```python
from build123d import *

# Parameters (mm, degrees)
F0_W     = 177.8
F0_H     = 228.6
F0_W_2   = 165.1
F0_H_2   = 215.9
F1_DEPTH = 279.4
F2_R     = 12.7
F2_R_2   = 38.829729
F3_DEPTH = 254
F4_R     = 17.145
F5_DEPTH = 254
F6_DEPTH = 25.4


with BuildPart() as f1:
    # F0 (on Top) → F1 (new body)
    with BuildSketch(Plane.XY):
        Rectangle(F0_W, F0_H)
        Rectangle(F0_W_2, F0_H_2, mode=Mode.SUBTRACT)
    extrude(amount=F1_DEPTH)

    # F2 (on Front) → F3 (cut)
    with BuildSketch(Plane.XZ):
        with Locations((0, 80.557629)):
            Circle(F2_R)
        with Locations((0, 161.839798)):
            Circle(F2_R_2)
    extrude(amount=F3_DEPTH, mode=Mode.SUBTRACT)

    # F4 (on Right) → F5 (cut)
    with BuildSketch(Plane.YZ):
        with Locations((0, 101.838969)):
            Circle(F4_R)
    extrude(amount=F5_DEPTH, mode=Mode.SUBTRACT)

    # F0 (on Top) → F6 (join)
    with BuildSketch(Plane.XY):
        Rectangle(F0_W_2, F0_H_2)
    extrude(amount=F6_DEPTH)


solid = f1.part
```
The model under review builds one solid part; all positions refer to its coordinate system, in mm. A direction names the side the tool comes from. Round coordinates to 2 decimals unless told otherwise and drop trailing zeros. Loops run counter-clockwise (first coordinate to the right, second up) from the corner with the lowest first, then second, coordinate; pieces in that order, holes last. Notation, with made-up numbers: (3.25, 28) -> (62.25, 28) arc R12 cw to (62.25, 48) -> close; hole circle Ø9 at (72, -7.5). An arc over 180 degrees is marked (long way). Answer in a Markdown table with one row per item.
1) Tool access review of faces 1 (the flat face through (-1, -114.3, 107)), 2 (the cylindrical face through (-2.75, -111.08, 68.16)), 3 (the flat face through (-1, -107.95, 122)): name each direction out of +Z, -Z, +X, -X, +Y, -Y from which nothing blocks a thin tool from reaching the whole face with its end or side.
Taken from the geometry:
| item | result |
|---|---|
| face 1 | +Z, -Z, +X, -X, -Y |
| face 2 | -Y |
| face 3 | +Z |
2) Draft analysis for pull direction X (two halves, no side actions). For faces 4 (the flat face through (-88.9, -2, 138)), 5 (the cylindrical face through (85.68, -2.23, 118.84)), 6 (the flat face through (-1, 107.95, 151)), state which applies: pulls with the +X half, pulls with the -X half, needs draft (parallel to the pull), parting line crosses it, or undercut.
Taken from the geometry:
| item | result |
|---|---|
| face 4 | pulls with the -X half |
| face 5 | needs draft |
| face 6 | undercut |
3) Consider section A-A, the plane y = 0. Write out the cut boundary in (x, z).
Taken from the geometry:
| item | result |
|---|---|
| outline | (-88.9, 0) -> (88.9, 0) -> (88.9, 84.69) -> (82.55, 84.69) -> (82.55, 25.4) -> (-82.55, 25.4) -> (-82.55, 279.4) -> (-88.9, 279.4) -> close; (82.55, 118.98) -> (88.9, 118.98) -> (88.9, 279.4) -> (82.55, 279.4) -> close |
4) Wall thickness on line 1 along Z through (x, y) = (0, -112.25); line 2 along X through (y, z) = (-8.5, 225); line 3 along Y through (x, z) = (15, 237): over which ranges is each line inside the solid? List them lowest first.
Taken from the geometry:
| item | result |
|---|---|
| line 1 | z = 0 to 67.86, 93.26 to 123.01, 200.67 to 279.4 |
| line 2 | x = -88.9 to -82.55, 82.55 to 88.9 |
| line 3 | y = -114.3 to -107.95, 107.95 to 114.3 |
5) Consider section C-C, the plane z = 219.5. Write out the cut boundary in (x, y).
Taken from the geometry:
| item | result |
|---|---|
| outline | (-88.9, -114.3) -> (88.9, -114.3) -> (88.9, 114.3) -> (-88.9, 114.3) -> close; hole (-82.55, -107.95) -> (82.55, -107.95) -> (82.55, 107.95) -> (-82.55, 107.95) -> close |
6) For pin 1 Ø1 at (x, z) = (-19.5, 149.5) entering from -Y; pin 2 Ø2 at (x, y) = (-60, 39) entering from +Z, all flat-tipped, find the tip position at first contact; note any pin that passes through.
Taken from the geometry:
| item | result |
|---|---|
| pin 1 | stops at y = 107.95 |
| pin 2 | stops at z = 25.4 |
7) Consider section B-B, the plane x = 0. Write out the cut boundary in (y, z).
Taken from the geometry:
| item | result |
|---|---|
| outline | (-114.3, 0) -> (114.3, 0) -> (114.3, 279.4) -> (107.95, 279.4) -> (107.95, 25.4) -> (-107.95, 25.4) -> (-107.95, 67.86) -> (-114.3, 67.86) -> close; (-114.3, 93.26) -> (-107.95, 93.26) -> (-107.95, 123.01) -> (-114.3, 123.01) -> close; (-114.3, 200.67) -> (-107.95, 200.67) -> (-107.95, 279.4) -> (-114.3, 279.4) -> close |
8) Consider section D-D, the plane x = -49. Write out the cut boundary in (y, z), plus the area to 3 significant figures.
Taken from the geometry:
| item | result |
|---|---|
| outline | (-114.3, 0) -> (114.3, 0) -> (114.3, 279.4) -> (107.95, 279.4) -> (107.95, 25.4) -> (-107.95, 25.4) -> (-107.95, 279.4) -> (-114.3, 279.4) -> close |
| area | 9,030 mm² |
